Autodesk Inventor part; units mm, degrees
ref_plane "YZ Plane" through (0, 0, 0) normal (1, 0, 0) x (0, 1, 0)
ref_plane "XZ Plane" through (0, 0, 0) normal (0, 1, 0) x (-1, 0, 0)
ref_plane "XY Plane" through (0, 0, 0) normal (0, 0, 1) x (1, 0, 0)
sketch "Sketch1" plane through (0, 0, 0) normal (1, 0, 0) x (0, 1, 0)
  line L0 (0, 0) -> (20, 0)
  line L1 (20, 0) -> (20, -20)
  line L2 (20, -20) -> (0, -20)
  line L3 (0, -20) -> (0, 0)
  dimension "d0" = 20
  dimension "d1" = 20
extrude "Extrusion1" add sketch "Sketch1" along normal blind 2
sketch "Sketch3" plane through (0, 20, 0) normal (0, 1, 0) x (1, 0, 0)
  circle A0 centre (7.75, 10) radius 7.75
  line L0 (2, 20) -> (2, 0)
  line L1 (2, 0) -> (10.1308, 2.6248)
  line L2 (2, 20) -> (10.1308, 17.3752)
  circle A1 centre (7.75, 10) radius 1.75
  line L3 (0, 20) -> (0, 0)
  dimension "d11" = 15.5
  dimension "d12" = 3.5
extrude "Extrusion3" add sketch "Sketch3" against normal blind 2 contours A0 L0 | A0 L0 L2 | L1 L0 A0 picked at (3.3333, 10)
chamfer "Chamfer3" distance 7 angle 45 1 edges at (2, 18, -10)
fillet "Fillet1" radius 2 4 edges at (1, 20, 0) (1, 0, 0) (1, 20, -20) (1, 0, -20)
sketch "Sketch4" plane through (0, 18, 0) normal (0, -1, 0) x (1, 0, 0)
  arc A0 (9, -11.2247) -> (9, -8.7753) centre (7.75, -10) ccw
  circle A1 centre (7.75, -10) radius 4.5
  point P0 (0, 0)
  dimension "d22" = 9
extrude "Extrusion4" cut sketch "Sketch4" along normal blind 6
properties part number "ChargingArm - FlatPlateBracket" material "ABS Plastic"
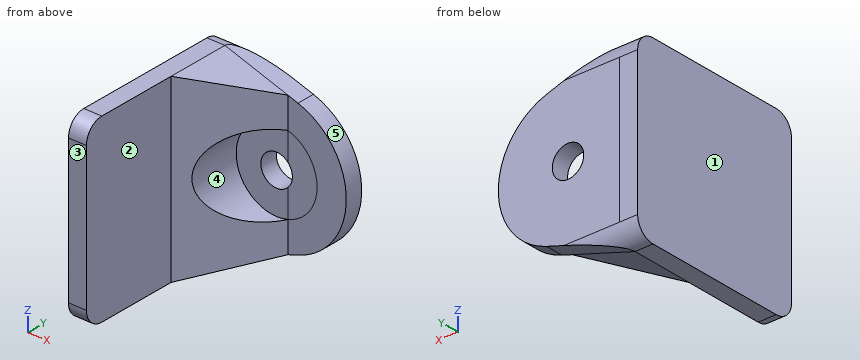
Here's how the part is built. I have some questions about the finished solid (model axes, mm). Face numbers are marked on the shaded views. A direction names the side the tool comes from. Round coordinates to 2 decimals unless told otherwise and drop trailing zeros. Order: outer loops, then holes, each group sorted by start corner. A loop starts at its lowest first (then second) coordinate and runs counter-clockwise, first axis right, second up. Notation, with made-up numbers: M 39.25,-20 L 84.25,-20 A23 cw 84.25,-5 Z; hole C 38.25,28.5 d2. An arc over 180 degrees is marked long. Return JSON: item names as keys, results as strings. Group by question number.
1. If we section it at C-C on y = 13.5: List the corners of the cut face in (x, z) for me, then the cut area to 3 significant figures.
2. On a 3-axis mill with a long thin cutter (end or side, diameter ignored), from which of +Z, -Z, +X, -X, +Y, -Y can I reach the whole of each face in a straight line? I mean the marked faces 1 and 2. Say none if no direction works.
3. If we section it at A-A on z = -10: List the corners of the cut face in (x, y) for me, then the cut area to 3 significant figures.
4. I'm going to push flat-ended pins straight in: pin 1 Ø7 at (x, z) = (7.75, -10) entering from -Y; pin 2 Ø3 at (x, y) = (4.5, 2.5) entering from -Z; pin 3 Ø3 at (y, z) = (10, -11.5) entering from +X; pin 4 Ø1 at (y, z) = (15.5, -2.5) entering from +X. Where does each tip first touch, or does it pass through?
5. If we mould it in two halves opening along Z, with no side actions, what happens to the marked faces 3, 4 and 5? For each: pulls with the +Z half, pulls with the -Z half, needs draft (parallel to the pull), parting line crosses it, or undercut.
6. Please list where these lines run through material, in increasing order: probe 1 along X at (y, z) = (15.8, -10); probe 2 along X at (y, z) = (8.5, -9.5); probe 3 along Y at (x, z) = (4.5, -12).
7. If we section it at D-D on z = -7: List the corners of the cut face in (x, y) for me.
8. If we section it at B-B on x = 8.5: List the corners of the cut face in (y, z) for me, then the cut area to 3 significant figures.
Reply:
{
 "1": {"outline": "M 0,-20 L 2,-20 L 4.5,-19.19 L 4.5,-13.11 A4.5 cw 4.5,-6.89 L 4.5,-0.81 L 2,0 L 0,0 Z", "area": "82.6 mm^2"},
 "2": {"face 1": "+Z, -Z, -X, +Y, -Y", "face 2": "+Z, -Z, +X, -Y"},
 "3": {"outline": "M 0,0 L 2,0 L 2,11 L 3.25,12.25 L 3.25,18 L 6,18 L 6,20 L 0,20 Z; M 9.5,18 L 15.5,18 L 15.5,20 L 9.5,20 Z", "area": "68.0 mm^2"},
 "4": {"pin 1": "y = 18", "pin 2": "through", "pin 3": "x = 2.5", "pin 4": "x = 7"},
 "5": {"face 3": "needs draft", "face 4": "undercut", "face 5": "parting line crosses it"},
 "6": {"probe 1": "0 to 3.25", "probe 2": "0 to 2", "probe 3": "18 to 20"},
 "7": {"outline": "M 0,0 L 2,0 L 2,11 L 4.4,13.4 L 4.4,18 L 14.9,18 L 14.9,20 L 0,20 Z"},
 "8": {"outline": "M 17.5,-17.9 L 20,-17.9 L 20,-11.58 L 18,-11.58 L 18,-14.44 L 17.5,-14.44 Z; M 17.5,-5.56 L 18,-5.56 L 18,-8.42 L 20,-8.42 L 20,-2.1 L 17.5,-2.1 Z", "area": "28.7 mm^2"}
}
